from build123d import *

# Parameters (mm, degrees)
BOSS_EXTRUDE1_DEPTH     = 10
SKETCH2_R               = 2
CUT_EXTRUDE1_DEPTH      = 131.192165663
LPATTERN2_COUNT         = 2
LPATTERN2_PITCH         = 8
CUT_EXTRUDE2_DEPTH      = 73.327380707
CUT_EXTRUDE2_DEPTH_BACK = 73.327380707
SKETCH3_R               = 2.5


with BuildPart() as part:
    # Sketch1 → Boss-Extrude1 (new, symmetric)
    with BuildSketch(Plane.XY):
        with BuildLine():
            Line((-57.5, 0), (57.5, 0))
            ThreePointArc((57.5, 0), (61.035533906, 1.464466094), (62.5, 5))
            Line((62.5, 5), (62.5, 35))
            Line((62.5, 35), (57.5, 35))
            Line((57.5, 35), (57.5, 10))
            ThreePointArc((57.5, 10), (56.035533906, 6.464466094), (52.5, 5))
            Line((52.5, 5), (-52.5, 5))
            ThreePointArc((-52.5, 5), (-56.035533906, 6.464466094), (-57.5, 10))
            Line((-57.5, 10), (-57.5, 35))
            Line((-57.5, 35), (-62.5, 35))
            Line((-62.5, 35), (-62.5, 5))
            ThreePointArc((-62.5, 5), (-61.035533906, 1.464466094), (-57.5, 0))
        make_face()
    extrude(amount=BOSS_EXTRUDE1_DEPTH, both=True)

    # Sketch2 → Cut-Extrude1 (cut, symmetric)
    with BuildSketch(Plane(origin=(62.5, 0, 0), x_dir=(0, 0, -1), z_dir=(1, 0, 0))):
        with Locations((0, 20)):
            Circle(SKETCH2_R)
    cut_extrude1 = extrude(amount=CUT_EXTRUDE1_DEPTH, both=True, mode=Mode.SUBTRACT)

    # LPattern2: Cut-Extrude1 ×2
    with Locations(*[(0, i * LPATTERN2_PITCH, 0) for i in range(1, LPATTERN2_COUNT)]):
        add(cut_extrude1, mode=Mode.SUBTRACT)

    # Sketch3 → Cut-Extrude2 (cut, two sides: drawn at the far end of the back side and taken through both)
    with BuildSketch(Plane.XZ.offset(-CUT_EXTRUDE2_DEPTH_BACK)):
        Circle(SKETCH3_R)
        with Locations((-10, 0)):
            Circle(SKETCH3_R)
        with Locations((-20, 0)):
            Circle(SKETCH3_R)
        with Locations((-30, 0)):
            Circle(SKETCH3_R)
        with Locations((-40, 0)):
            Circle(SKETCH3_R)
        with Locations(Location((-50, 0, 0), (0, 0, 180))):
            Circle(SKETCH3_R)
        with Locations((10, 0)):
            Circle(SKETCH3_R)
        with Locations((20, 0)):
            Circle(SKETCH3_R)
        with Locations((30, 0)):
            Circle(SKETCH3_R)
        with Locations((40, 0)):
            Circle(SKETCH3_R)
        with Locations((50, 0)):
            Circle(SKETCH3_R)
    extrude(amount=CUT_EXTRUDE2_DEPTH + CUT_EXTRUDE2_DEPTH_BACK, mode=Mode.SUBTRACT)


solid = part.part
Work out the finished part from the listing and answer in its coordinate system (mm). A direction names the side the tool comes from. Coordinates: 2 decimals unless noted, no trailing zeros. Write each loop counter-clockwise with the first axis right and the second up, starting at its lowest first coordinate (ties: lowest second). Pieces come first, ordered by that corner, then holes.
1. For a pull along Y with two mould halves and no side action, classify faces 3 (the flat face through (-1, 0, 5)), 4 (the cylindrical face through (60, 26, 0)), 5 (the cylindrical face through (-22.5, 2.5, 0.1)) as +Y half, -Y half, draft (parallel to the pull), parting line (faces both ways), or undercut.
Results list:
face 3: -Y half
face 4: undercut
face 5: draft
2. The part is cut by section C-C, the plane y = 28. Write down the section's boundary in (x, z), and give its area (3 significant figures).
Results list:
outline: (-62.5, -10) - (-57.5, -10) - (-57.5, -2) - (-62.5, -2) - close; (-62.5, 2) - (-57.5, 2) - (-57.5, 10) - (-62.5, 10) - close; (57.5, -10) - (62.5, -10) - (62.5, -2) - (57.5, -2) - close; (57.5, 2) - (62.5, 2) - (62.5, 10) - (57.5, 10) - close
area: 160 mm2
3. The part is cut by section A-A, the plane y = 14.5. Write down the section's boundary in (x, z), and give its area (3 significant figures).
Results list:
outline: (-62.5, -10) - (-57.5, -10) - (-57.5, 10) - (-62.5, 10) - close; (57.5, -10) - (62.5, -10) - (62.5, 10) - (57.5, 10) - close
area: 200 mm2
4. Consider line 1 along X through (y, z) = (17, 7.5); line 2 along Z through (x, y) = (20, 1.75); line 3 along Y through (x, z) = (-61.1, 0). Determine where each line is inside the solid, lowest interval first.
Results list:
line 1: x = -62.5 to -57.5, 57.5 to 62.5
line 2: z = -10 to -2.5, 2.5 to 10
line 3: y = 1.53 to 18, 22 to 26, 30 to 35
5. The part is cut by section B-B, the plane x = -40. Write down the section's boundary in (y, z).
Results list:
outline: (0, -10) - (5, -10) - (5, -2.5) - (0, -2.5) - close; (0, 2.5) - (5, 2.5) - (5, 10) - (0, 10) - close
6. The part is cut by section D-D, the plane x = -5. Write down the section's boundary in (y, z), and give its area (3 significant figures).
Results list:
outline: (0, -10) - (5, -10) - (5, 10) - (0, 10) - close
area: 100 mm2
7. Flat-ended cylindrical pins translate along their axes: pin 1 (6.5 mm diameter, centred on x = 20, z = 0, fed in from +Y); pin 2 (6.5 mm diameter, centred on x = 50, z = 0, fed in from +Y). Find the tip coordinate at first contact, or state that the pin passes through.
Results list:
pin 1: stops at y = 5
pin 2: stops at y = 5.06
8. For faces 1 (the flat face through (0, 3, 10)), 2 (the flat face through (57.5, 23, 0)), determine the directions among +Z, -Z, +X, -X, +Y, -Y from which every point of the face is accessible in a straight line to the end or side of a thin tool.
Results list:
face 1: +Z, +X, -X, +Y, -Y
face 2: +Z, -Z, +Y
